from build123d import *

# Parameters (mm, degrees)
FILLET003_R = 1
FILLET004_R = 1


with BuildPart() as part:
    # Sketch002 → Revolution001 (revolve)
    with BuildSketch(Plane.XZ):
        Polygon((1.75, 33.5), (8.5, 33.5), (8.5, 15.5), (7, 15.5), (7, 32), (1.75, 32), align=None)
    revolve(axis=Axis((0, 0, 0), (0, 0, 1)))

    # Fillet003
    fillet003_edges = [part.edges().sort_by_distance(p)[0] for p in [
        (-8.5, 0, 15.5),
    ]]
    fillet(fillet003_edges, radius=FILLET003_R)

    # Fillet004
    fillet004_edges = [part.edges().sort_by_distance(p)[0] for p in [
        (-7, 0, 32),
    ]]
    fillet(fillet004_edges, radius=FILLET004_R)


solid = part.part
Part model, mm, in its own coordinate system. A direction names the side the tool comes from. Coordinates: 2 decimals unless noted, no trailing zeros. Write each loop counter-clockwise with the first axis right and the second up, starting at its lowest first coordinate (ties: lowest second). Pieces come first, ordered by that corner, then holes. Notation, with made-up numbers: M 70,23.25 L 128,23.25 A13 cw 128,39.25 Z; hole C -16.75,41.5 d7. An arc over 180 degrees is marked long. Return JSON: item names as keys, results as strings.
1. Pull direction Y, two halves, no side cores. Call faces 1 (the face through (7, 2, 15.5)), 2 (the face through (4.57, 7.167, 24.881)), 3 (the face through (1.617, -0.67, 32.76)): pulls with the +Y half, pulls with the -Y half, needs draft (parallel to the pull), parting line crosses it, or undercut.
Determined:
{"face 1": "needs draft", "face 2": "parting line crosses it", "face 3": "undercut"}
2. Flat gauge pins, fed straight in: pin 1 Ø1.5 at (x, z) = (-5.5, 27.5) entering from -Y; pin 2 Ø3 at (y, z) = (-4.5, 29) entering from +X; pin 3 Ø3 at (x, z) = (5.5, 31.5) entering from -Y; pin 4 Ø3 at (x, y) = (0, 0) entering from -Z. Where does each tip first touch, or does it go through?
Determined:
{"pin 1": "y = -7.05", "pin 2": "x = 7.95", "pin 3": "y = -7.5", "pin 4": "through"}
3. Probe L1, parallel to Y at x = 0, z = 33; L2, parallel to Y at x = 0, z = 17.5; L3, parallel to Z at x = -1.25, y = 4.5. List the from-to ranges inside material, lowest first.
Determined:
{"L1": "-8.5 to -1.75, 1.75 to 8.5", "L2": "-8.5 to -7, 7 to 8.5", "L3": "32 to 33.5"}
4. 3-axis set-ups, long thin cutter, end or side, ignore diameter. For faces 4 (the face through (-1.4, 1.4, 32)), 5 (the face through (-2, 0, 33.5)): which of +Z, -Z, +X, -X, +Y, -Y reach the whole face in a straight line?
Determined:
{"face 4": "-Z", "face 5": "+Z, +X, -X, +Y, -Y"}
5. Saw through at C-C, the plane z = 25. Write the cut outline in (x, y).
Determined:
{"outline": "C 0,0 d17; hole C 0,0 d14"}
6. Saw through at A-A, the plane x = 0. Write the cut outline in (y, z), then the cut area to 4 significant figures.
Determined:
{"outline": "M -8.5,16.5 A1 ccw -7.5,15.5 L -7,15.5 L -7,31 A1 cw -6,32 L -1.75,32 L -1.75,33.5 L -8.5,33.5 Z; M 1.75,32 L 6,32 A1 cw 7,31 L 7,15.5 L 7.5,15.5 A1 ccw 8.5,16.5 L 8.5,33.5 L 1.75,33.5 Z", "area": "69.75 mm²"}
